Design review of the part built by this model. Coordinates are the model's own, in mm. Round coordinates to 2 decimals unless told otherwise and drop trailing zeros. Loops run counter-clockwise (first coordinate to the right, second up) from the corner with the lowest first, then second, coordinate; pieces in that order, holes last. Notation, with made-up numbers: (13.25, 26.25) -> (59.25, 26.25) arc R23 ccw to (59.25, 44.25) -> close; hole circle Ø1 at (41, 67.5). An arc over 180 degrees is marked (long way). Answer as CSV lines item,"result". Start each with the question number.
(1) Draft analysis for pull direction X (two halves, no side actions). For faces 1 (the face through (26, 6, 93)), 2 (the face through (0, 6, 125)), state which applies: +X half, -X half, draft (parallel to the pull), parting line (faces both ways), or undercut.
(2) Take a section at B-B, the plane z = 204.5. Write out the cut boundary in (x, y), and give its area (3 significant figures).
(3) Take a section at C-C, the plane y = 4.5. State how many separate pieces and enclosed holes the cut face has, and give its area (3 significant figures).
(4) Take a section at A-A, the plane z = 103. Write out the cut boundary in (x, y).
(5) To check wall thickness, follow line 1 (X direction, y = 2, z = 135.5); line 2 (X direction, y = 9.5, z = 215.5); line 3 (X direction, y = 5.75, z = 126). State the ranges of each line that lie inside material, in increasing order. Write a range as from..to.
from build123d import *

# Parameters (mm, degrees)
CROQUIS1_W              = 349.003555023
CROQUIS1_H              = 246
SALIENTE_EXTRUIR1_DEPTH = 12


with BuildPart() as part:
    # Croquis1 → Saliente-Extruir1 (new body)
    with BuildSketch(Plane(origin=(0, 0, 0), x_dir=(1, 0, 0), z_dir=(0, 1, 0))):
        with Locations((174.501777512, -123)):
            Rectangle(CROQUIS1_W, CROQUIS1_H)
        with BuildLine():
            Line((17.121320344, -173), (23.878679656, -173))
            ThreePointArc((23.878679656, -173), (26, -173), (26, -170.878679656))
            Line((26, -170.878679656), (26, -136.121320344))
            ThreePointArc((26, -136.121320344), (26, -134), (23.878679656, -134))
            Line((23.878679656, -134), (17.121320344, -134))
            ThreePointArc((17.121320344, -134), (15, -134), (15, -136.121320344))
            Line((15, -136.121320344), (15, -170.878679656))
            ThreePointArc((15, -170.878679656), (15, -173), (17.121320344, -173))
        make_face(mode=Mode.SUBTRACT)
        with BuildLine():
            Line((46, -149.757359313), (46, -93.058131736))
            ThreePointArc((46, -93.058131736), (45.941048988, -90.937630668), (48.061550056, -90.878679656))
            Line((48.061550056, -90.878679656), (54.878679656, -90.878679656))
            ThreePointArc((54.878679656, -90.878679656), (57, -90.878679656), (57, -93))
            Line((57, -93), (57, -149.757359313))
            ThreePointArc((57, -149.757359313), (57, -151.878679656), (54.878679656, -151.878679656))
            Line((54.878679656, -151.878679656), (48.121320344, -151.878679656))
            ThreePointArc((48.121320344, -151.878679656), (46, -151.878679656), (46, -149.757359313))
        make_face(mode=Mode.SUBTRACT)
        with BuildLine():
            Line((17.121320344, -112), (23.878679656, -112))
            ThreePointArc((23.878679656, -112), (26, -112), (26, -109.878679656))
            Line((26, -109.878679656), (26, -75.121320344))
            ThreePointArc((26, -75.121320344), (26, -73), (23.878679656, -73))
            Line((23.878679656, -73), (17.121320344, -73))
            ThreePointArc((17.121320344, -73), (15, -73), (15, -75.121320344))
            Line((15, -75.121320344), (15, -109.878679656))
            ThreePointArc((15, -109.878679656), (15, -112), (17.121320344, -112))
        make_face(mode=Mode.SUBTRACT)
        with BuildLine():
            Line((26, -231.878679656), (26, -197.121320344))
            ThreePointArc((26, -197.121320344), (26, -195), (23.878679656, -195))
            Line((23.878679656, -195), (17.121320344, -195))
            ThreePointArc((17.121320344, -195), (15, -195), (15, -197.121320344))
            Line((15, -197.121320344), (15, -231.878679656))
            ThreePointArc((15, -231.878679656), (15, -234), (17.121320344, -234))
            Line((17.121320344, -234), (23.878679656, -234))
            ThreePointArc((23.878679656, -234), (26, -234), (26, -231.878679656))
        make_face(mode=Mode.SUBTRACT)
        with BuildLine():
            Line((17.121320344, -51), (23.878679656, -51))
            ThreePointArc((23.878679656, -51), (26, -51), (26, -48.878679656))
            Line((26, -48.878679656), (26, -14.121320344))
            ThreePointArc((26, -14.121320344), (26, -12), (23.878679656, -12))
            Line((23.878679656, -12), (17.121320344, -12))
            ThreePointArc((17.121320344, -12), (15, -12), (15, -14.121320344))
            Line((15, -14.121320344), (15, -48.878679656))
            ThreePointArc((15, -48.878679656), (15, -51), (17.121320344, -51))
        make_face(mode=Mode.SUBTRACT)
        with BuildLine():
            Line((331.88223468, -234), (325.124875367, -234))
            ThreePointArc((325.124875367, -234), (323.003555023, -234), (323.003555023, -231.878679656))
            Line((323.003555023, -231.878679656), (323.003555023, -197.121320344))
            ThreePointArc((323.003555023, -197.121320344), (323.003555023, -195), (325.124875367, -195))
            Line((325.124875367, -195), (331.88223468, -195))
            ThreePointArc((331.88223468, -195), (334.003555023, -195), (334.003555023, -197.121320344))
            Line((334.003555023, -197.121320344), (334.003555023, -231.878679656))
            ThreePointArc((334.003555023, -231.878679656), (334.003555023, -234), (331.88223468, -234))
        make_face(mode=Mode.SUBTRACT)
        with BuildLine():
            Line((325.124875367, -173), (331.88223468, -173))
            ThreePointArc((331.88223468, -173), (334.003555023, -173), (334.003555023, -170.878679656))
            Line((334.003555023, -170.878679656), (334.003555023, -136.121320344))
            ThreePointArc((334.003555023, -136.121320344), (334.003555023, -134), (331.88223468, -134))
            Line((331.88223468, -134), (325.124875367, -134))
            ThreePointArc((325.124875367, -134), (323.003555023, -134), (323.003555023, -136.121320344))
            Line((323.003555023, -136.121320344), (323.003555023, -170.878679656))
            ThreePointArc((323.003555023, -170.878679656), (323.003555023, -173), (325.124875367, -173))
        make_face(mode=Mode.SUBTRACT)
        with BuildLine():
            Line((325.124875367, -112), (331.88223468, -112))
            ThreePointArc((331.88223468, -112), (334.003555023, -112), (334.003555023, -109.878679656))
            Line((334.003555023, -109.878679656), (334.003555023, -75.121320344))
            ThreePointArc((334.003555023, -75.121320344), (334.003555023, -73), (331.88223468, -73))
            Line((331.88223468, -73), (325.124875367, -73))
            ThreePointArc((325.124875367, -73), (323.003555023, -73), (323.003555023, -75.121320344))
            Line((323.003555023, -75.121320344), (323.003555023, -109.878679656))
            ThreePointArc((323.003555023, -109.878679656), (323.003555023, -112), (325.124875367, -112))
        make_face(mode=Mode.SUBTRACT)
        with BuildLine():
            Line((325.124875367, -51), (331.88223468, -51))
            ThreePointArc((331.88223468, -51), (334.003555023, -51), (334.003555023, -48.878679656))
            Line((334.003555023, -48.878679656), (334.003555023, -14.121320344))
            ThreePointArc((334.003555023, -14.121320344), (334.003555023, -12), (331.88223468, -12))
            Line((331.88223468, -12), (325.124875367, -12))
            ThreePointArc((325.124875367, -12), (323.003555023, -12), (323.003555023, -14.121320344))
            Line((323.003555023, -14.121320344), (323.003555023, -48.878679656))
            ThreePointArc((323.003555023, -48.878679656), (323.003555023, -51), (325.124875367, -51))
        make_face(mode=Mode.SUBTRACT)
        with BuildLine():
            Line((303.003555023, -149.757359313), (303.003555023, -93))
            ThreePointArc((303.003555023, -93), (303.003555023, -90.878679656), (300.88223468, -90.878679656))
            Line((300.88223468, -90.878679656), (294.124875367, -90.878679656))
            ThreePointArc((294.124875367, -90.878679656), (292.003555023, -90.878679656), (292.003555023, -93))
            Line((292.003555023, -93), (292.003555023, -149.757359313))
            ThreePointArc((292.003555023, -149.757359313), (292.003555023, -151.878679656), (294.124875367, -151.878679656))
            Line((294.124875367, -151.878679656), (300.88223468, -151.878679656))
            ThreePointArc((300.88223468, -151.878679656), (303.003555023, -151.878679656), (303.003555023, -149.757359313))
        make_face(mode=Mode.SUBTRACT)
    extrude(amount=SALIENTE_EXTRUIR1_DEPTH)


solid = part.part
The answers:
1,face 1,"undercut"
1,face 2,"-X half"
2,outline,"(0, 0) -> (15, 0) -> (15, 12) -> (0, 12) -> close; (26, 0) -> (323, 0) -> (323, 12) -> (26, 12) -> close; (334, 0) -> (349, 0) -> (349, 12) -> (334, 12) -> close"
2,area,"3,920 mm²"
3,separate pieces,"1"
3,enclosed holes,"10"
3,area,"81,000 mm²"
4,outline,"(0, 0) -> (15, 0) -> (15, 12) -> (0, 12) -> close; (26, 0) -> (46, 0) -> (46, 12) -> (26, 12) -> close; (57, 0) -> (292, 0) -> (292, 12) -> (57, 12) -> close; (303, 0) -> (323, 0) -> (323, 12) -> (303, 12) -> close; (334, 0) -> (349, 0) -> (349, 12) -> (334, 12) -> close"
5,line 1,"0..14.63, 26.37..46, 57..292, 303..322.63, 334.38..349"
5,line 2,"0..15, 26..323, 334..349"
5,line 3,"0..46, 57..292, 303..349"
